Autodesk Inventor part; units mm, degrees
ref_plane "YZ Plane" through (0, 0, 0) normal (1, 0, 0) x (0, 1, 0)
ref_plane "XZ Plane" through (0, 0, 0) normal (0, 1, 0) x (-1, 0, 0)
ref_plane "XY Plane" through (0, 0, 0) normal (0, 0, 1) x (1, 0, 0)
sketch "Sketch1" plane through (0, 0, 0) normal (0, 0, 1) x (1, 0, 0)
  circle A0 centre (0, 0) radius 5
  line L0 (2.9551, -5) -> (-2.8526, -5.0592)
  line L1 (-2.8526, -5.0592) -> (-5.8077, -0.0592)
  line L2 (-5.8077, -0.0592) -> (-2.9551, 5)
  line L3 (-2.9551, 5) -> (2.8526, 5.0592)
  line L4 (2.8526, 5.0592) -> (5.8077, 0.0592)
  line L5 (5.8077, 0.0592) -> (2.9551, -5)
  dimension "d0" = 10
extrude "Extrusion1" add sketch "Sketch1" along normal blind 5 contours A0 | L0 L1 L2 L3 L4 L5
sketch "Sketch2" plane through (0, 0, 5) normal (0, 0, 1) x (1, 0, 0)
  circle A0 centre (0, 0) radius 2.5
  dimension "d3" = 5
extrude "Extrusion2" cut sketch "Sketch2" against normal blind 12.5
thread "Thread1"
properties part number "Nut"
Build history of the part. All positions in model axes, mm. Give positions to 0.01 mm unless a question says otherwise; leave off trailing zeros. Order: outer loops, then holes, each group sorted by start corner. A loop starts at its lowest first (then second) coordinate and runs counter-clockwise, first axis right, second up. Notation, with made-up numbers: M -38.75,-4 L 1.25,-4 A11 cw 1.25,10 Z; hole C -14,85 d11. An arc over 180 degrees is marked long. Write item = value, one per line. Start each with the question number.
(1) Probe L1, parallel to Y at x = -1.5, z = 2; L2, parallel to X at y = 1.75, z = 1.3; L3, parallel to Y at x = -2.25, z = 2.1. List the from-to ranges inside material, lowest first. Write a range as [from, to].
(2) Slice it at D-D on x = 4. Write the cut outline in (y, z).
(3) Slice it at B-B on z = 1.7. Write the cut outline in (x, y), plus the area to 3 significant figures.
(4) Slice it at A-A on y = -0.25. Write the cut outline in (x, z).
(5) Slice it at C-C on x = 0. Write the cut outline in (y, z).
(6) Two-plate mould, pull along X, no slides. Class faces 1 (the flat face through (2.5, 1.2, 5)), 2 (the cylindrical face through (-0.54, -2.44, 2.54)), 3 (the flat face through (-4.31, -2.59, 2.46)), 4 (the flat face through (4.31, 2.59, 2.46)): released by +X, released by -X, zero draft, split by the parting line, or undercut.
Responses:
q1.L1 = [-5.05, -2], [2, 5.01]
q1.L2 = [-4.79, -1.79], [1.79, 4.81]
q1.L3 = [-5.05, -1.09], [1.09, 5.01]
q2.outline = M -3.15,0 L 3.12,0 L 3.12,5 L -3.15,5 Z
q3.outline = M -5.81,-0.06 L -2.85,-5.06 L 2.96,-5 L 5.81,0.06 L 2.85,5.06 L -2.96,5 Z; hole C 0,0 d5
q3.area = 68.0 mm2
q4.outline = M -5.69,0 L -2.49,0 L -2.49,5 L -5.69,5 Z; M 2.49,0 L 5.63,0 L 5.63,5 L 2.49,5 Z
q5.outline = M -5.03,0 L -2.5,0 L -2.5,5 L -5.03,5 Z; M 2.5,0 L 5.03,0 L 5.03,5 L 2.5,5 Z
q6.face_1 = zero draft
q6.face_2 = undercut
q6.face_3 = released by -X
q6.face_4 = released by +X
